CAD build for the part. Positions are in the model's coordinates, mm. A direction names the side the tool comes from. Give positions to 0.01 mm unless a question says otherwise; leave off trailing zeros. Order: outer loops, then holes, each group sorted by start corner. A loop starts at its lowest first (then second) coordinate and runs counter-clockwise, first axis right, second up.
```python
from build123d import *

# Parameters (mm, degrees)
F0_R     = 4.36
F1_DEPTH = 5
F2_SIZE2 = 0.288675
F2_SIZE  = 0.5
F4_DEPTH = 2.5
F5_R     = 2.5
F6_DEPTH = 15
F7_SIZE  = 0.5


with BuildPart() as f1:
    # F0 (on Right) → F1 (new body)
    with BuildSketch(Plane.YZ):
        Circle(F0_R)
    extrude(amount=-F1_DEPTH)

    # F2
    f2_edges = [f1.edges().sort_by_distance(p)[0] for p in [
        (0, -4.36, 0),
        (-5, -4.36, 0),
    ]]
    chamfer(f2_edges, length=F2_SIZE, length2=F2_SIZE2)

    # F3 (on face) → F4 (cut)
    with BuildSketch(Plane.YZ):
        Polygon((0, -2.364249), (2.0475, -1.182125), (2.0475, 1.182125), (0, 2.364249), (-2.0475, 1.182125), (-2.0475, -1.182125), align=None)
    extrude(amount=-F4_DEPTH, mode=Mode.SUBTRACT)

    # F5 (on face) → F6 (join)
    with BuildSketch(Plane(origin=(-5, 0, 0), x_dir=(0, -1, 0), z_dir=(-1, 0, 0))):
        Circle(F5_R)
    extrude(amount=F6_DEPTH)

    # F7
    f7_edges = [f1.edges().sort_by_distance(p)[0] for p in [
        (-20, 2.5, 0),
    ]]
    chamfer(f7_edges, length=F7_SIZE)


solid = f1.part
```
Item 1: Wall check: L1, parallel to X at y = 2, z = -2.5; L2, parallel to Z at x = -1.25, y = -1.25; L3, parallel to Z at x = -1, y = -1.5. Give the ranges that are in metal, low to high.
Item 2: Drop flat-ended pins along their axis: pin 1 Ø1 at (x, z) = (-3, -3) entering from +Y; pin 2 Ø4 at (x, z) = (-3, 1) entering from -Y; pin 3 Ø1.5 at (x, y) = (-9, -0.5) entering from +Z. Give the stop position or say it passes through.
Item 3: Slice it at A-A (z = 0). Give the cut face in (x, y), and give its area (3 significant figures).
Item 4: Slice it at B-B (x = -16.5). Give the cut face in (y, z), and give its area (3 significant figures).
Item 5: Two-plate mould, pull along Z, no slides. Class faces 1 (the face through (-12.15, 0.54, -2.44)), 2 (the face through (-1.232, 1.038, 1.765)), 3 (the face through (0, -1, 2)): released by +Z, released by -Z, zero draft, split by the parting line, or undercut.
Item 6: Tool access for faces 4 (the face through (-5, -2, -2)), 5 (the face through (-1, 2.047, 0)), 6 (the face through (-20, 0, 0)): list every direction of +Z, -Z, +X, -X, +Y, -Y with a clear straight run to the whole face (end or side of a thin tool).
A:
1. L1: x = -5 to 0
1. L2: z = -4.18 to -1.64, 1.64 to 4.18
1. L3: z = -4.09 to -1.5, 1.5 to 4.09
2. pin 1: stops at y = 3.57
2. pin 2: stops at y = -4.36
2. pin 3: stops at z = 2.5
3. outline: (-20, -2) - (-19.5, -2.5) - (-5, -2.5) - (-5, -4.07) - (-4.5, -4.36) - (-0.5, -4.36) - (0, -4.07) - (0, -2.05) - (-2.5, -2.05) - (-2.5, 2.05) - (0, 2.05) - (0, 4.07) - (-0.5, 4.36) - (-4.5, 4.36) - (-5, 4.07) - (-5, 2.5) - (-19.5, 2.5) - (-20, 2) - close
3. area: 108 mm2
4. outline: circle Ø5 at (0, 0)
4. area: 19.6 mm2
5. face 1: split by the parting line
5. face 2: undercut
5. face 3: zero draft
6. face 4: -X
6. face 5: +X
6. face 6: +Z, -Z, -X, +Y, -Y
